```python
from build123d import *

# Parameters (mm, degrees)
BOX034_W          = 10
BOX034_H          = 2.5
BOX034_DEPTH      = 10
CYLINDER029_R     = 10.2
CYLINDER029_DEPTH = 10
BOX035_W          = 30
BOX035_H          = 30
BOX035_DEPTH      = 3


with BuildPart() as cube034:
    # Box034 → Box034 (new body)
    with BuildSketch(Plane(origin=(85.6, 163.75, -5), x_dir=(1, 0, 0), z_dir=(0, 0, 1))):
        with Locations((5, 1.25)):
            Rectangle(BOX034_W, BOX034_H)
    extrude(amount=BOX034_DEPTH)


with BuildPart() as obj1:
    # Cylinder029 → Cylinder029 (new body)
    with BuildSketch(Plane(origin=(85, 165, -5), x_dir=(1, 0, 0), z_dir=(0, 0, 1))):
        Circle(CYLINDER029_R)
    extrude(amount=CYLINDER029_DEPTH)

    # Fusion001: union Cube034
    add(cube034.part)


with BuildPart() as obj1_1:
    # Fusion001 placement: moved
    add(obj1.part.moved(Location((130, 50, 0))))


with BuildPart() as obj2:
    # Box035 → Box035 (new body)
    with BuildSketch(Plane(origin=(200, 200, 0), x_dir=(1, 0, 0), z_dir=(0, 0, 1))):
        with Locations((15, 15)):
            Rectangle(BOX035_W, BOX035_H)
    extrude(amount=BOX035_DEPTH)

    # Cut044: cut obj1
    add(obj1_1.part, mode=Mode.SUBTRACT)


solid = obj2.part
```
The listing builds one solid part. Answer for the finished solid, in the listing's coordinates (mm). Coordinates: 2 decimals unless noted, no trailing zeros. Write each loop counter-clockwise with the first axis right and the second up, starting at its lowest first coordinate (ties: lowest second). Pieces come first, ordered by that corner, then holes.
Q1. The mould has two halves that part along X. Classify faces 1 (the flat face through (225.6, 215, 1)), 2 (the flat face through (205, 219, 3)), 3 (the flat face through (230, 215, 1)): released by +X, released by -X, zero draft, split by the parting line, or undercut.
Returned:
face 1: undercut
face 2: zero draft
face 3: released by +X
Q2. Section A-A, the plane x = 215 is taken. Write down the section's boundary in (y, z).
Returned:
outline: (200, 0) - (204.8, 0) - (204.8, 3) - (200, 3) - close; (225.2, 0) - (230, 0) - (230, 3) - (225.2, 3) - close
Q3. Section B-B, the plane y = 215 is taken. Write down the section's boundary in (x, z).
Returned:
outline: (200, 0) - (204.8, 0) - (204.8, 3) - (200, 3) - close; (225.6, 0) - (230, 0) - (230, 3) - (225.6, 3) - close
Q4. Find the intervals of material crossed by line 1 along Y through (x, z) = (215, 1.3); line 2 along X through (y, z) = (215, 1.65); line 3 along X through (y, z) = (221.5, 0.2), in increasing order.
Returned:
line 1: y = 200 to 204.8, 225.2 to 230
line 2: x = 200 to 204.8, 225.6 to 230
line 3: x = 200 to 207.14, 222.86 to 230
Q5. Given P1, Ø12, axis at x = 215, y = 215, coming from the -Z side; P2, Ø6, axis at x = 224.5, y = 212, coming from the +Z side, each flat-ended and moving along its own axis, determine where each tip first touches the part or whether it passes through.
Returned:
P1: passes through
P2: stops at z = 3
Q6. Section C-C, the plane z = 2.25 is taken. Write down the section's boundary in (x, y), then the cut area to 3 significant figures.
Returned:
outline: (200, 200) - (230, 200) - (230, 230) - (200, 230) - close; hole (225.12, 213.75) - (225.6, 213.75) - (225.6, 216.25) - (225.12, 216.25) arc R10.2 ccw (long way) to start
area: 572 mm2
